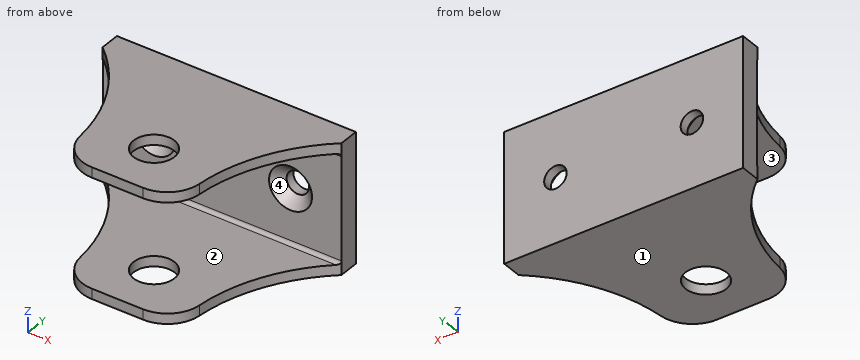
from build123d import *

# Parameters (mm, degrees)
SZKIC1_R                                 = 6
DODANIE_WYCI_GNI_CIE1_DEPTH              = 38
SZKIC2_W                                 = 70
SZKIC2_H                                 = 32
WYTNIJ_WYCI_GNI_CIE1_DEPTH               = 43
ZAOKR_GLENIE1_R                          = 1
POG_BIENIE_STO_KOWE_POD_M6_RUB_Z_2_COUNT = 2
POG_BIENIE_STO_KOWE_POD_M6_RUB_Z_2_PITCH = 40


with BuildPart() as part:
    # Szkic1 → Dodanie-wyciągnięcie1 (new body)
    with BuildSketch(Plane.XY):
        with BuildLine():
            Line((0, 48.768640881), (0, 42.89244343))
            ThreePointArc((0, 42.89244343), (12.102069866, 27.737632724), (17.527104902, 9.1178213))
            ThreePointArc((17.527104902, 9.1178213), (20.736146372, 2.623625993), (27.488116936, 0))
            Line((27.488116936, 0), (42.511883064, 0))
            ThreePointArc((42.511883064, 0), (49.263853628, 2.623625993), (52.472895098, 9.1178213))
            ThreePointArc((52.472895098, 9.1178213), (57.897930134, 27.737632724), (70, 42.89244343))
            Line((70, 42.89244343), (70, 48.768640881))
            Line((70, 48.768640881), (0, 48.768640881))
        make_face()
        with Locations((35, 15)):
            Circle(SZKIC1_R, mode=Mode.SUBTRACT)
    extrude(amount=DODANIE_WYCI_GNI_CIE1_DEPTH)

    # Szkic2 → Wytnij-wyciągnięcie1 (cut)
    with BuildSketch(Plane.XZ):
        with Locations((35, 19)):
            Rectangle(SZKIC2_W, SZKIC2_H)
    extrude(amount=-WYTNIJ_WYCI_GNI_CIE1_DEPTH, mode=Mode.SUBTRACT)

    # Zaokrąglenie1
    zaokr_glenie1_edges = [part.edges().sort_by_distance(p)[0] for p in [
        (35, 43, 35),
        (35, 43, 3),
    ]]
    fillet(zaokr_glenie1_edges, radius=ZAOKR_GLENIE1_R)

    # Szkic5 → Pogłębienie stożkowe pod M6 Śrubę z łbem soczewkowym1 (revolve, cut)
    with BuildSketch(Plane(origin=(15, 43, 19), x_dir=(0, 0, -1), z_dir=(1, 0, 0))):
        Polygon((0, 0), (0, 5.768640881), (3.3, 5.768640881), (3.3, 3), (6.3, 0), align=None)
    pog_bienie_sto_kowe_pod_m6_rub_z_bem = revolve(axis=Axis((15, 36.65, 19), (0, 1, 0)), mode=Mode.SUBTRACT)

    # Pog_bienie sto_kowe pod M6 _rub_ z _ 2: Pogłębienie stożkowe pod M6 Śrubę z łbem soczewkowym1 ×2
    with Locations(*[(i * POG_BIENIE_STO_KOWE_POD_M6_RUB_Z_2_PITCH, 0, 0) for i in range(1, POG_BIENIE_STO_KOWE_POD_M6_RUB_Z_2_COUNT)]):
        add(pog_bienie_sto_kowe_pod_m6_rub_z_bem, mode=Mode.SUBTRACT)


solid = part.part
Read the model definition and answer for the solid it produces. Units are mm, in the model's axes. Face numbers are marked on the shaded views. A direction names the side the tool comes from. Coordinates: 2 decimals unless noted, no trailing zeros. Loops run counter-clockwise (first coordinate to the right, second up) from the corner with the lowest first, then second, coordinate; pieces in that order, holes last.
Q1. The part is cut by section B-B on z = 19. Write down the section's boundary in (x, y), and give its area (3 significant figures).
Q2. The part is cut by section D-D on x = 15. Write down the section's boundary in (y, z).
Q3. The mould has two halves that part along X. Classify the marked faces 3 and 4: +X half, -X half, draft (parallel to the pull), parting line (faces both ways), or undercut.
Q4. Which of the six approach directions +Z, -Z, +X, -X, +Y, -Y give full straight-line access (tool end or side, diameter ignored) to the marked faces 1 and 2?
Q5. The part is cut by section A-A on x = 35. Write down the section's boundary in (y, z).
Q6. This flat-tipped pin is pushed along its axis until it touches: pin 1 Ø9 at (x, z) = (26.5, 11.5) entering from -Y. Where does it stop, or does it pass through?
Q7. The part is cut by section C-C on y = 13. Write down the section's boundary in (x, z).
Q8. Consider probe 1 along X at (y, z) = (47, 19); probe 2 along Z at (x, y) = (45, 31); probe 3 along Y at (x, z) = (35, 36.05). Determine where each line is inside the solid, lowest interval first.
Results below:
1. outline: (0, 43) - (8.7, 43) - (11.7, 46) - (11.7, 48.77) - (0, 48.77) - close; (18.3, 46) - (21.3, 43) - (48.7, 43) - (51.7, 46) - (51.7, 48.77) - (18.3, 48.77) - close; (58.3, 46) - (61.3, 43) - (70, 43) - (70, 48.77) - (58.3, 48.77) - close
1. area: 310 mm2
2. outline: (20.98, 0) - (48.77, 0) - (48.77, 15.7) - (46, 15.7) - (43, 12.7) - (43, 4) arc R1 cw to (42, 3) - (20.98, 3) - close; (20.98, 35) - (42, 35) arc R1 cw to (43, 34) - (43, 25.3) - (46, 22.3) - (48.77, 22.3) - (48.77, 38) - (20.98, 38) - close
3. face 3: draft
3. face 4: undercut
4. face 1: -Z, +X, -X, +Y, -Y
4. face 2: +X, -X, -Y
5. outline: (0, 0) - (9, 0) - (9, 3) - (0, 3) - close; (0, 35) - (9, 35) - (9, 38) - (0, 38) - close; (21, 0) - (48.77, 0) - (48.77, 38) - (21, 38) - (21, 35) - (42, 35) arc R1 cw to (43, 34) - (43, 4) arc R1 cw to (42, 3) - (21, 3) - close
6. pin 1: stops at y = 43
7. outline: (17.03, 0) - (29.34, 0) - (29.34, 3) - (17.03, 3) - close; (17.03, 35) - (29.34, 35) - (29.34, 38) - (17.03, 38) - close; (40.66, 0) - (52.97, 0) - (52.97, 3) - (40.66, 3) - close; (40.66, 35) - (52.97, 35) - (52.97, 38) - (40.66, 38) - close
8. probe 1: x = 0 to 11.7, 18.3 to 51.7, 58.3 to 70
8. probe 2: z = 0 to 3, 35 to 38
8. probe 3: y = 0 to 9, 21 to 48.77
